Part model, mm, in its own coordinate system. A direction names the side the tool comes from. Round coordinates to 2 decimals unless told otherwise and drop trailing zeros. Loops run counter-clockwise (first coordinate to the right, second up) from the corner with the lowest first, then second, coordinate; pieces in that order, holes last. Notation, with made-up numbers: M -7,54.25 L 30,54.25 A34 ccw 30,90.25 Z; hole C 10.25,81.25 d3. An arc over 180 degrees is marked long. Write each question's results on one line, items separated by ' | '.
from build123d import *

# Parameters (mm, degrees)
F1_DEPTH = 20
F2_W     = 8
F2_H     = 84.6575228283
F5_DEPTH = 40.001
F6_R     = 2.6
F7_DEPTH = 12.815167995
F8_SIZE  = 5


with BuildPart() as f1:
    # F0 (on Front) → F1 (new body, symmetric)
    with BuildSketch(Plane.XZ):
        Polygon((-7.8440168473, 89.6575228283), (0, 0), (5.0190991877, 0), (-2.3874743419, 84.6575228283), (32.1559831527, 84.6575228283), (32.1559831527, 89.6575228283), align=None)
    extrude(amount=F1_DEPTH, both=True)

    # F2 (on face) → F3 (join, up to the next surface of F1)
    with BuildSketch(Plane.YZ.offset(32.1559831527)):
        with Locations((0, 42.3287614141)):
            Rectangle(F2_W, F2_H)
    extrude(until=Until.NEXT, dir=(-1, 0, 0))

    # F4 (on face) → F5 (cut, through all)
    with BuildSketch(Plane.XZ.offset(20)):
        Polygon((32.1559831527, 84.6575228283), (5.0190991877, 0), (32.1559831527, 0), align=None)
    extrude(amount=-F5_DEPTH, mode=Mode.SUBTRACT)

    # F6 (on face) → F7 (cut, through all)
    with BuildSketch(Plane(origin=(4.9809734905, 0, 0.4357787137), x_dir=(0, 1, 0), z_dir=(0.9961946981, 0, 0.0871557427))):
        with Locations((12.5, 69.5625566824)):
            Circle(F6_R)
        with Locations((12.5, 19.5625566824)):
            Circle(F6_R)
        with Locations((-12.5, 69.5625566824)):
            Circle(F6_R)
        with Locations((-12.5, 19.5625566824)):
            Circle(F6_R)
    extrude(amount=-F7_DEPTH, mode=Mode.SUBTRACT)

    # F8
    f8_edges = [f1.edges().sort_by_distance(p)[0] for p in [
        (32.155983, -20, 87.157523),
        (32.155983, 20, 87.157523),
    ]]
    chamfer(f8_edges, length=F8_SIZE)


solid = f1.part
Item 1: Band-saw the part on B-B on y = 11. Give the cut face in (x, z), and give its area (3 significant figures).
Filled sheet:
outline: M -7.84,89.66 L -6.25,71.41 L -1.27,71.85 L -2.39,84.66 L 32.16,84.66 L 32.16,89.66 Z; M -5.88,67.18 L -1.89,21.6 L 3.09,22.04 L -0.9,67.62 Z; M -1.52,17.37 L 0,0 L 5.02,0 L 3.46,17.81 Z | area: 581 mm^2
Item 2: Wall check: L1, parallel to Z at x = 29, y = -7; L2, parallel to Y at x = 20.5, z = 49.5; L3, parallel to X at y = 13.5, z = 46.5. Give the ranges that are in metal, low to high.
Filled sheet:
L1: 84.66 to 89.66 | L2: -4 to 4 | L3: -4.07 to 0.95
Item 3: Band-saw the part on D-D on z = 52.5. Give the cut face in (x, y).
Filled sheet:
outline: M -4.59,-20 L 0.43,-20 L 0.43,-4 L 21.85,-4 L 21.85,4 L 0.43,4 L 0.43,20 L -4.59,20 Z
Item 4: Drop flat-ended pins along their axis: P1, Ø1, axis at y = 3, z = 36, coming from the +X side; P2, Ø6, axis at y = -1, z = 26, coming from the -X side; P3, Ø5, axis at x = 5, z = 49, coming from the +Y side. Give the stop position or say it passes through.
Filled sheet:
P1: x = 16.72 | P2: x = -2.54 | P3: y = 4
Item 5: Band-saw the part on C-C on x = 10.5. Give the cut face in (y, z), and give its area (3 significant figures).
Filled sheet:
outline: M -20,84.66 L -4,84.66 L -4,17.1 L 4,17.1 L 4,84.66 L 20,84.66 L 20,89.66 L -20,89.66 Z | area: 740 mm^2
Item 6: Which spindle directions (+Z, -Z, +X, -X, +Y, -Y) get a long thin tool onto all of the face, cutting with end or side? Do faces 4 (the flat face through (11, 4, 61)), 5 (the cylindrical face through (-3.451, -10.098, 68.527)), 6 (the flat face through (15, -12, 84.658)). Say none if no direction does.
Filled sheet:
face 4: +X, +Y | face 5: none | face 6: +X, -Y
Item 7: Two-plate mould, pull along Z, no slides. Class faces 1 (the flat face through (12, 0, 89.658)), 2 (the flat face through (1.368, 11.888, 41.736)), 3 (the flat face through (18.777, -0.056, 42.921)): +Z half, -Z half, draft (parallel to the pull), parting line (faces both ways), or undercut.
Filled sheet:
face 1: +Z half | face 2: undercut | face 3: -Z half
Item 8: Band-saw the part on A-A on y = -0.5. Give the cut face in (x, z), and give its area (3 significant figures).
Filled sheet:
outline: M -7.84,89.66 L 0,0 L 5.02,0 L 32.16,84.66 L 32.16,89.66 Z | area: 2,090 mm^2
